from build123d import *

# Parameters (mm, degrees)
SKETCH_2_W          = 29
SKETCH_2_H          = 19
EXTRUDE_1_DEPTH     = 2
SKETCH_3_W          = 24
SKETCH_3_H          = 10
EXTRUDE_2_DEPTH     = 16
SKETCH_4_W          = 21
SKETCH_4_H          = 13
CUT_EXTRUDE_1_DEPTH = 8.5
SKETCH_5_R          = 2.5
EXTRUDE_3_DEPTH     = 3


with BuildPart() as part:
    # 草图2 → 凸台-拉伸1 (new body)
    with BuildSketch(Plane.XY):
        Rectangle(SKETCH_2_W, SKETCH_2_H)
    extrude(amount=EXTRUDE_1_DEPTH)

    # 草图3 → 凸台-拉伸2 (add)
    with BuildSketch(Plane(origin=(0, 0, 0), x_dir=(-1, 0, 0), z_dir=(0, 0, -1))):
        with Locations((0, -2.5)):
            Rectangle(SKETCH_3_W, SKETCH_3_H)
    extrude(amount=EXTRUDE_2_DEPTH)

    # 草图4 → 切除-拉伸1 (cut)
    with BuildSketch(Plane(origin=(0, 2.5, 0), x_dir=(1, 0, 0), z_dir=(0, 1, 0))):
        with Locations((0, 8)):
            Rectangle(SKETCH_4_W, SKETCH_4_H)
    extrude(amount=-CUT_EXTRUDE_1_DEPTH, mode=Mode.SUBTRACT)

    # 草图5 → 凸台-拉伸3 (add)
    with BuildSketch(Plane.XY.offset(2)):
        with Locations(Location((0, 0, 0), (0, 0, 180))):
            Circle(SKETCH_5_R)
    extrude(amount=EXTRUDE_3_DEPTH)


solid = part.part
Could you check a few things on this model? Use its own coordinates, in mm. A direction names the side the tool comes from. Give positions to 0.01 mm unless a question says otherwise; leave off trailing zeros. Loops run counter-clockwise (first coordinate to the right, second up) from the corner with the lowest first, then second, coordinate; pieces in that order, holes last. Notation, with made-up numbers: M -10,80 L -5,80 A34 ccw -5,119 Z; hole C 67.25,56.25 d6. An arc over 180 degrees is marked long. Answer as a JSON object with one key per item and string values.
Q1. For P1, Ø7, axis at y = -2.5, z = -5.5, coming from the +X side; P2, Ø2.5, axis at y = -0.5, z = -5.5, coming from the -X side; P3, Ø4, axis at x = 10, y = 5, coming from the +Z side, each with a flat end and sliding along its axis, tell me the tip position at first contact or that it passes through.
Values found:
{"P1": "stops at x = 12", "P2": "stops at x = -12", "P3": "stops at z = 2"}
Q2. Suppose I cut it at A-A, the plane y = -4.75. List the corners of the cut face in (x, z) for me.
Values found:
{"outline": "M -14.5,0 L -12,0 L -12,-16 L 12,-16 L 12,0 L 14.5,0 L 14.5,2 L -14.5,2 Z; hole M -10.5,-14.5 L 10.5,-14.5 L 10.5,-1.5 L -10.5,-1.5 Z"}
Q3. If we mould it in two halves opening along X, with no side actions, what happens to faces 1 (the flat face through (-10.5, -2, -8)), 2 (the flat face through (3, 0, 2)), 3 (the cylindrical face through (2.5, -0.1, 3.5))? For each: pulls with the +X half, pulls with the -X half, needs draft (parallel to the pull), parting line crosses it, or undercut.
Values found:
{"face 1": "undercut", "face 2": "needs draft", "face 3": "parting line crosses it"}
Q4. If I drill on probe 1 along X at (y, z) = (-3, -14); probe 2 along Z at (x, y) = (9, -3.5); probe 3 along Z at (x, y) = (-11.5, -1), over which ranges is the centre line in solid material (lowest first)? Write a range as [from, to].
Values found:
{"probe 1": "x = [-12, -10.5], [10.5, 12]", "probe 2": "z = [-16, -14.5], [-1.5, 2]", "probe 3": "z = [-16, 2]"}
Q5. For faces 4 (the flat face through (-12, -3, -8)), 5 (the flat face through (0, -2, -14.5)), 6 (the flat face through (12, -3, -8)), which set-ups out of +Z, -Z, +X, -X, +Y, -Y let a thin tool reach every point of the face, with its end or its side?
Values found:
{"face 4": "-Z, -X, +Y, -Y", "face 5": "+Y", "face 6": "-Z, +X, +Y, -Y"}
Q6. Suppose I cut it at B-B, the plane z = -4.5. List the corners of the cut face in (x, y) for me.
Values found:
{"outline": "M -12,-7.5 L 12,-7.5 L 12,2.5 L 10.5,2.5 L 10.5,-6 L -10.5,-6 L -10.5,2.5 L -12,2.5 Z"}
Q7. Suppose I cut it at D-D, the plane y = 0. List the corners of the cut face in (x, z) for me, plus the area to 3 significant figures.
Values found:
{"outline": "M -14.5,0 L -12,0 L -12,-16 L 12,-16 L 12,0 L 14.5,0 L 14.5,2 L 2.5,2 L 2.5,5 L -2.5,5 L -2.5,2 L -14.5,2 Z; hole M -10.5,-14.5 L 10.5,-14.5 L 10.5,-1.5 L -10.5,-1.5 Z", "area": "184 mm²"}
Q8. Suppose I cut it at C-C, the plane x = 0. List the corners of the cut face in (y, z) for me.
Values found:
{"outline": "M -9.5,0 L -7.5,0 L -7.5,-16 L 2.5,-16 L 2.5,-14.5 L -6,-14.5 L -6,-1.5 L 2.5,-1.5 L 2.5,0 L 9.5,0 L 9.5,2 L 2.5,2 L 2.5,5 L -2.5,5 L -2.5,2 L -9.5,2 Z"}
